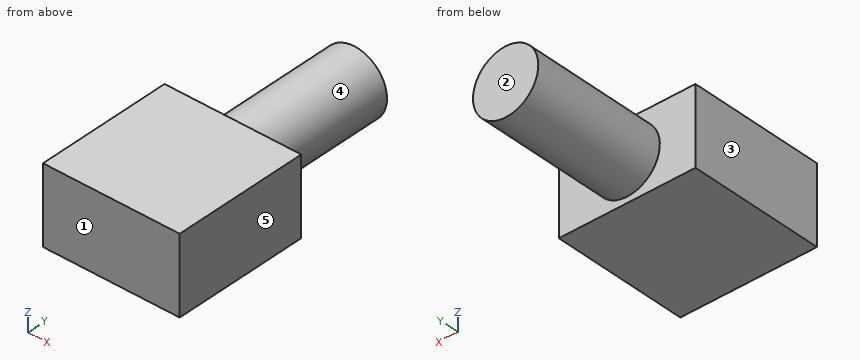
```python
from build123d import *

# Parameters (mm, degrees)
SKETCH_1_W          = 80
SKETCH_1_H          = 45
EXTRUDE_1_DEPTH     = 80
CUT_EXTRUDE_START   = -1
SKETCH_3_W          = 76
SKETCH_3_H          = 41
CUT_EXTRUDE_1_DEPTH = 68
CUT_EXTRUDE_1_DRAFT = -3
SKETCH_11_R         = 19.112902973
EXTRUDE_2_DEPTH     = 80


with BuildPart() as part:
    # 스케치1 → 보스-돌출1 (new body)
    with BuildSketch(Plane(origin=(0, 0, 0), x_dir=(1, 0, 0), z_dir=(0, 1, 0))):
        Rectangle(SKETCH_1_W, SKETCH_1_H)
    extrude(amount=EXTRUDE_1_DEPTH)


with BuildPart() as cut_extrude_1_tool:
    # 스케치3 → 컷-돌출1 (with draft: the straight prism first)
    with BuildSketch(Plane(origin=(0, 80, 0), x_dir=(1, 0, 0), z_dir=(0, 1, 0)).offset(CUT_EXTRUDE_START)):
        Rectangle(SKETCH_3_W, SKETCH_3_H)
    extrude(amount=-CUT_EXTRUDE_1_DEPTH)
    # 컷-돌출1: the draft: its side faces are tilted about the plane it starts from
    cut_extrude_1_sides = [cut_extrude_1_tool.faces().sort_by_distance(p)[0] for p in [
        (0, 45, 20.5),
        (38, 45, 0),
        (0, 45, -20.5),
        (-38, 45, 0),
    ]]
    draft(cut_extrude_1_sides, Plane(origin=(0, 80, 0), x_dir=(1, 0, 0), z_dir=(0, 1, 0)).offset(CUT_EXTRUDE_START), CUT_EXTRUDE_1_DRAFT)


with BuildPart() as part_1:
    add(part.part)

    # 컷-돌출1: cut by cut_extrude_1_tool
    add(cut_extrude_1_tool.part, mode=Mode.SUBTRACT)

    # 스케치11 → 보스-돌출2 (add)
    with BuildSketch(Plane(origin=(0, 80, 0), x_dir=(1, 0, 0), z_dir=(0, 1, 0))):
        with Locations(Location((0, 0, 0), (0, 0, 270))):
            Circle(SKETCH_11_R)
    extrude(amount=EXTRUDE_2_DEPTH)


solid = part_1.part
```
Source: CAD feature listing. Evaluate the final solid. Frame: model axes, mm. Face numbers are marked on the shaded views. A direction names the side the tool comes from. Round coordinates to 2 decimals unless told otherwise and drop trailing zeros. Write each loop counter-clockwise with the first axis right and the second up, starting at its lowest first coordinate (ties: lowest second). Pieces come first, ordered by that corner, then holes. Notation, with made-up numbers: M 72,79.5 L 112,79.5 A28 ccw 112,103.5 Z; hole C 24,73.25 d1. An arc over 180 degrees is marked long. Answer as a JSON object with one key per item and string values. Group by question number.
(1) Section query D-D on y = 118. Output: boundary loops of the cut face in (x, z).
(2) Ray query, line 1 (Y direction, x = 15.5, z = -13.5); line 2 (Y direction, x = -2.5, z = -9); line 3 (Z direction, x = -0.5, y = 53). Return the intervals inside material, ascending. Write a range as [from, to].
(3) Section query C-C on y = 14. Output: boundary loops of the cut face in (x, z).
(4) Section query B-B on x = -32. Output: boundary loops of the cut face in (y, z), then the cut area to 3 significant figures.
(5) Mould query, pull axis Y, two halves, no side actions, for the marked faces 1, 2 and 3. Classes: +Y half, -Y half, draft (parallel to the pull), parting line (faces both ways), or undercut.
(6) Section query A-A on z = 0. Output: boundary loops of the cut face in (x, y), then the cut area to 3 significant figures.
(7) First-contact query: pin 1 (4 mm diameter, centred on y = 89.5, z = 15.5, fed in from -X); pin 2 (12 mm diameter, centred on y = 119, z = -6.5, fed in from +X); pin 3 (10 mm diameter, centred on x = 9.5, y = 106.5, fed in from -Z). Flat tips, straight axial feed; report the tip coordinate or a pass-through.
(8) Reachability of the marked faces 4 and 5 from +Z, -Z, +X, -X, +Y, -Y: full face, straight path, thin tool, end or side. Return the list, or none.
Computed values:
{
 "1": {"outline": "C 0,0 d38.23"},
 "2": {"line 1": "[0, 11], [79, 80]", "line 2": "[0, 11], [79, 160]", "line 3": "[-22.5, -19.14], [19.14, 22.5]"},
 "3": {"outline": "M -40,-22.5 L 40,-22.5 L 40,22.5 L -40,22.5 Z; hole M -34.59,-17.09 L 34.59,-17.09 L 34.59,17.09 L -34.59,17.09 Z"},
 "4": {"outline": "M 0,-22.5 L 80,-22.5 L 80,22.5 L 0,22.5 Z; hole M 11,-16.94 L 79,-20.5 L 79,20.5 L 11,16.94 Z", "area": "1,050 mm^2"},
 "5": {"face 1": "-Y half", "face 2": "+Y half", "face 3": "draft"},
 "6": {"outline": "M -40,0 L 40,0 L 40,80 L 19.11,80 L 19.11,160 L -19.11,160 L -19.11,80 L -40,80 Z; hole M -38,79 L -34.44,11 L 34.44,11 L 38,79 Z", "area": "4,530 mm^2"},
 "7": {"pin 1": "x = -13.53", "pin 2": "x = 19.11", "pin 3": "z = -18.58"},
 "8": {"face 4": "+Y", "face 5": "+Z, -Z, +X, +Y, -Y"}
}
